```python
from build123d import *

# Parameters (mm, degrees)
F1_DEPTH = 86.106
F3_DEPTH = 58.928


with BuildPart() as f1:
    # F0 (on Top) → F1 (new body)
    with BuildSketch(Plane.XY):
        with BuildLine():
            Line((-119.3899347218, 81.5751131241), (-119.3899347218, 36.099622529))
            ThreePointArc((-119.3899347218, 36.099622529), (-119.0183715142, -12.8191604773), (-106.3290840641, 34.4266581107))
            Line((-106.3290840641, 34.4266581107), (-91.9901505113, 70.7625672221))
            Line((-91.9901505113, 70.7625672221), (-119.3899347218, 81.5751131241))
        make_face()
    extrude(amount=F1_DEPTH)

    # F2 (on face) → F3 (cut)
    with BuildSketch(Plane.XY.offset(86.106)):
        with BuildLine():
            Line((-106.3290840641, 34.4266581107), (-103.2862087041, 42.1375274103))
            ThreePointArc((-103.2862087041, 42.1375274103), (-114.2122343511, 31.8629620744), (-99.3326582188, 29.9806912638))
            ThreePointArc((-99.3326582188, 29.9806912638), (-102.6429075582, 32.4994648534), (-106.3290840641, 34.4266581107))
        make_face()
    extrude(amount=-F3_DEPTH, mode=Mode.SUBTRACT)


solid = f1.part
```
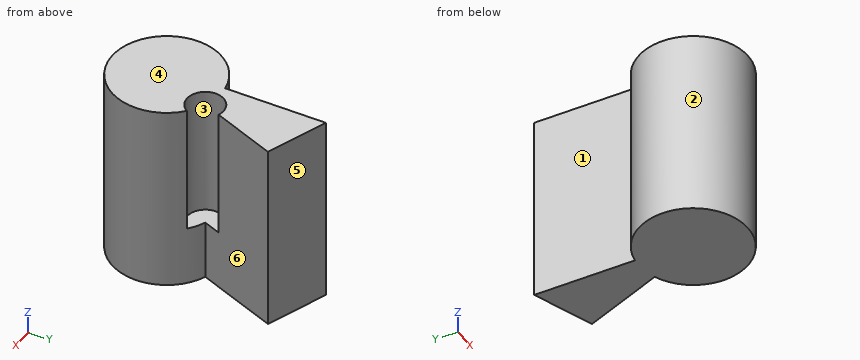
Work out the finished part from the listing and answer in its coordinate system (mm). Face numbers are marked on the shaded views. A direction names the side the tool comes from. Give positions to 0.01 mm unless a question says otherwise; leave off trailing zeros. Loops run counter-clockwise (first coordinate to the right, second up) from the corner with the lowest first, then second, coordinate; pieces in that order, holes last. Notation, with made-up numbers: (16.5, 74) -> (54.5, 74) arc R16 cw to (54.5, 82) -> close; hole circle Ø6 at (9, 28.5). An arc over 180 degrees is marked (long way). Put each result on its own line as item: value. Start each with the question number.
Item 1: Find the intervals of material crossed by L1, parallel to Y at x = -107, z = 68; L2, parallel to Y at x = -111, z = 32; L3, parallel to X at y = 62, z = 56, in increasing order. Write a range as [from, to].
Item 2: Which of the six approach directions +Z, -Z, +X, -X, +Y, -Y give full straight-line access (tool end or side, diameter ignored) to the marked faces 1, 2 and 3?
Item 3: The part is cut by section C-C (x = -134). Give the vertices of the cut face in (y, z).
Item 4: Each of these flat-tipped pins is pushed along its axis until it touches: P1, Ø17, axis at x = -104, y = 31, coming from the +Z side; P2, Ø1, axis at x = -128, z = 70, coming from the +Y side; P3, Ø5, axis at x = -108, z = 32, coming from the -Y side; P4, Ø1.5, axis at x = -117.5, z = 12, coming from the -Y side. Where does it stop, or does it pass through?
Item 5: The part is cut by section B-B (z = 57.5). Give the vertices of the cut face in (x, y).
Item 6: The mould has two halves that part along Y. Classify the marked faces 4, 5 and 6: released by +Y, released by -Y, zero draft, split by the parting line, or undercut.
Item 7: The part is cut by section D-D (y = -2). Give the vertices of the cut face in (x, z).
Item 8: The part is cut by section A-A (y = 32). Give the vertices of the cut face in (x, z).
Answers below:
1. L1: [-11.37, 26.16], [42.69, 76.69]
1. L2: [-12.53, 27.58], [41.27, 78.26]
1. L3: [-119.39, -95.45]
2. face 1: +Z, -Z, -X, +Y
2. face 2: +Z, -Z
2. face 3: +Z
3. outline: (-5.1, 0) -> (28.43, 0) -> (28.43, 86.11) -> (-5.1, 86.11) -> close
4. P1: z = 86.11
4. P2: y = 33.45
4. P3: y = -12.43
4. P4: y = -13
5. outline: (-119.39, 36.1) arc R24.68 ccw (long way) to (-99.33, 29.98) arc R8.29 cw (long way) to (-103.29, 42.14) -> (-91.99, 70.76) -> (-119.39, 81.58) -> close
6. face 4: zero draft
6. face 5: released by +Y
6. face 6: undercut
7. outline: (-136.44, 0) -> (-95.33, 0) -> (-95.33, 86.11) -> (-136.44, 86.11) -> close
8. outline: (-129.88, 0) -> (-101.89, 0) -> (-101.89, 27.18) -> (-114.26, 27.18) -> (-114.26, 86.11) -> (-129.88, 86.11) -> close
